Here's the drawing with two shaded views (mm, measured from the low corner). I have some questions. Give positions to 0.01 mm unless a question says otherwise; leave off trailing zeros. Write each loop counter-clockwise with the first axis right and the second up, starting at its lowest first coordinate (ties: lowest second). Pieces come first, ordered by that corner, then holes.
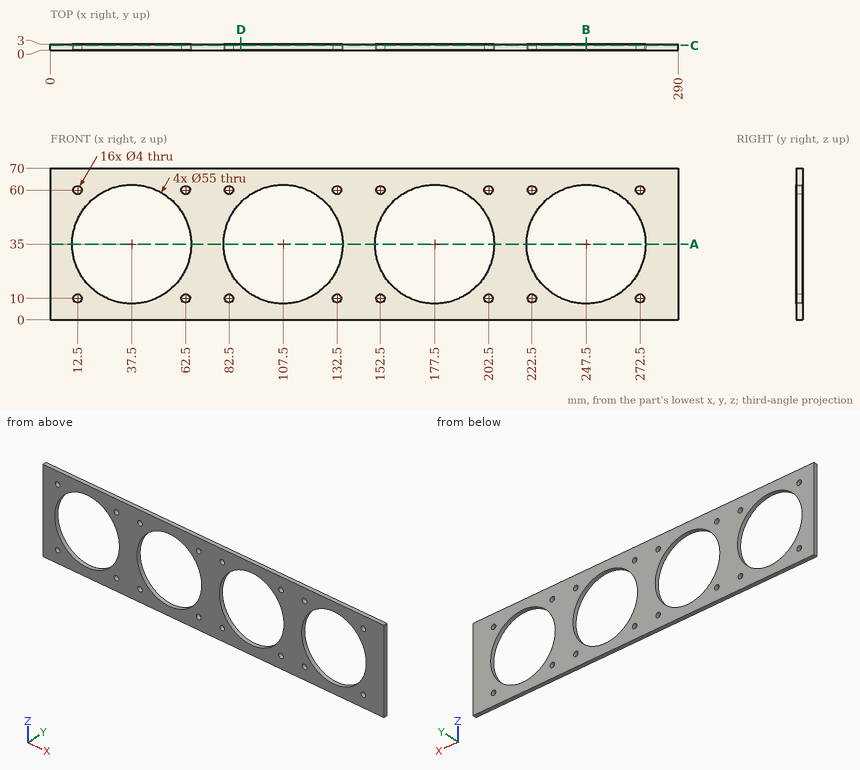
(1) Imagine slicing it at A-A, the plane z = 35. Write out the boundary of the cut face in (x, y).
Returned:
outline: (0, 0) - (10, 0) - (10, 3) - (0, 3) - close; (65, 0) - (80, 0) - (80, 3) - (65, 3) - close; (135, 0) - (150, 0) - (150, 3) - (135, 3) - close; (205, 0) - (220, 0) - (220, 3) - (205, 3) - close; (275, 0) - (290, 0) - (290, 3) - (275, 3) - close
(2) If I drill on L1, parallel to X at y = 1.3, z = 30; L2, parallel to X at y = 2.15, z = 35; L3, parallel to Z at x = 177, y = 0.25, over which ranges is the centre line in solid material (lowest first)?
Returned:
L1: x = 0 to 10.46, 64.54 to 80.46, 134.54 to 150.46, 204.54 to 220.46, 274.54 to 290
L2: x = 0 to 10, 65 to 80, 135 to 150, 205 to 220, 275 to 290
L3: z = 0 to 7.5, 62.5 to 70
(3) Will this pin go through, and if not, where does the flat tip stop? P1, Ø2.5, axis at x = 222.5, z = 60, coming from the -Y side.
Returned:
P1: passes through
(4) Imagine slicing it at D-D, the plane x = 88. Write out the boundary of the cut face in (y, z).
Returned:
outline: (0, 0) - (3, 0) - (3, 15.61) - (0, 15.61) - close; (0, 54.39) - (3, 54.39) - (3, 70) - (0, 70) - close
(5) Imagine slicing it at C-C, the plane y = 2.4. Give the number of separate pieces and of enclosed holes in the cut face, plus the area to 3 significant figures.
Returned:
separate pieces: 1
enclosed holes: 20
area: 10,600 mm2
(6) Imagine slicing it at B-B, the plane x = 247.5. Write out the boundary of the cut face in (y, z), plus the area to 3 significant figures.
Returned:
outline: (0, 0) - (3, 0) - (3, 7.5) - (0, 7.5) - close; (0, 62.5) - (3, 62.5) - (3, 70) - (0, 70) - close
area: 45.0 mm2
